The drawing under review shows one solid part. Ordinate dimensions are in mm from its lowest x, y, z. A direction names the side the tool comes from. Coordinates: 2 decimals unless noted, no trailing zeros. Write each loop counter-clockwise with the first axis right and the second up, starting at its lowest first coordinate (ties: lowest second). Pieces come first, ordered by that corner, then holes.
Q1. Insertion check: pin 1 (10 mm diameter, centred on x = 38.5, z = 21, fed in from -Y); pin 2 (6 mm diameter, centred on y = 11, z = 19.1, fed in from -X); pin 3 (4.5 mm diameter, centred on y = 79, z = 19.1, fed in from -X); pin 4 (4 mm diameter, centred on x = 94, z = 28.5, fed in from -Y). Each pin has a flat end and moves straight along its axis. Give the tip position at first contact, or say it passes through.
Q2. Take a section at D-D (y = 11). Give the boundary of the cut face in (x, z).
Q3. Take a section at A-A (y = 32). Give the boundary of the cut face in (x, z).
Q4. Mouldability with a two-part tool opening along X and no side actions: class the marked faces 3, 4 and 5 as pulls with the +X half, pulls with the -X half, needs draft (parallel to the pull), parting line crosses it, or undercut.
Q5. Take a section at C-C (z = 19.1). State how many separate pieces and enclosed holes the cut face has, and give its area (3 significant figures).
Q6. Take a section at B-B (x = 75). Give the boundary of the cut face in (y, z).
Q7. Machinability: for the marked faces 1 and 2, which of the approach directions +Z, -Z, +X, -X, +Y, -Y give a long, thin tool a straight path to every point of the face, cutting with its end or side? Answer none if there is none.
Q8. For probe 1 along X at (y, z) = (32, 17.5); probe 2 along Y at (x, z) = (2.3, 19.1); probe 3 along Y at (x, z) = (1, 19) (1 decimal), list the stretches that pass through material, from the lowest coordinate up.
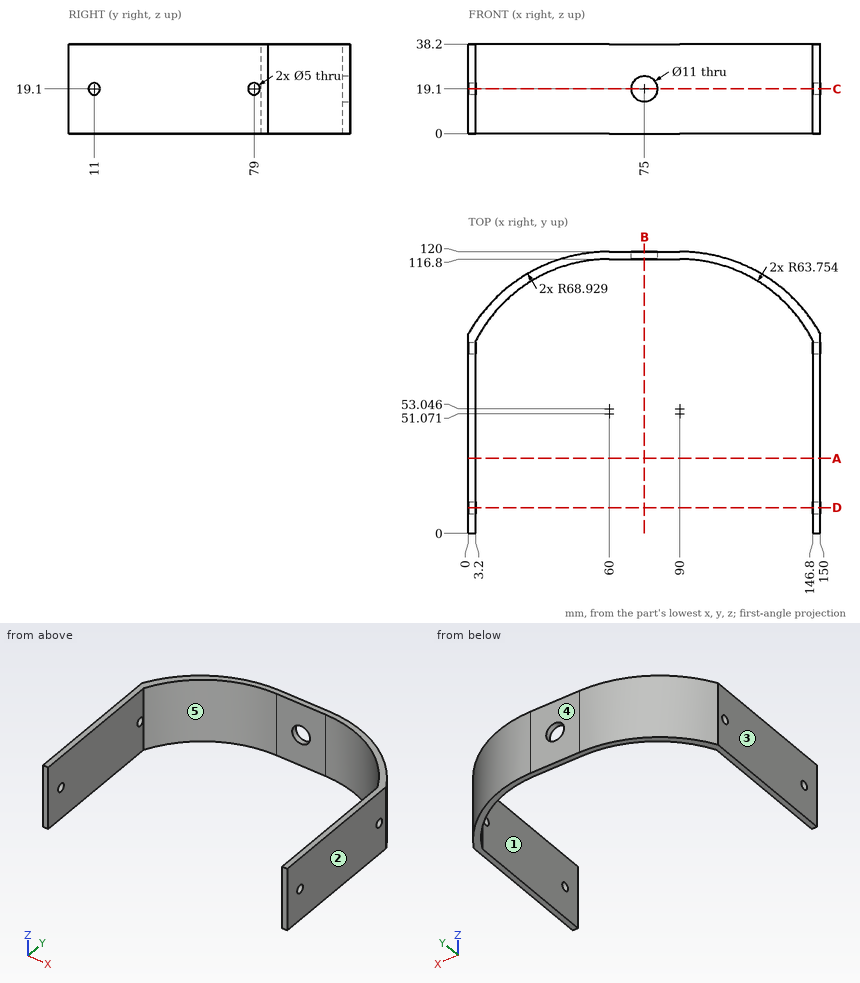
Response:
1. pin 1: stops at y = 111.03
1. pin 2: stops at x = 0
1. pin 3: passes through
1. pin 4: stops at y = 116.52
2. outline: (0, 0) - (3.2, 0) - (3.2, 16.6) - (0, 16.6) - close; (0, 21.6) - (3.2, 21.6) - (3.2, 38.2) - (0, 38.2) - close; (146.8, 0) - (150, 0) - (150, 16.6) - (146.8, 16.6) - close; (146.8, 21.6) - (150, 21.6) - (150, 38.2) - (146.8, 38.2) - close
3. outline: (0, 0) - (3.2, 0) - (3.2, 38.2) - (0, 38.2) - close; (146.8, 0) - (150, 0) - (150, 38.2) - (146.8, 38.2) - close
4. face 3: pulls with the -X half
4. face 4: needs draft
4. face 5: undercut
5. separate pieces: 6
5. enclosed holes: 0
5. area: 1,040 mm2
6. outline: (116.8, 0) - (120, 0) - (120, 13.6) - (116.8, 13.6) - close; (116.8, 24.6) - (120, 24.6) - (120, 38.2) - (116.8, 38.2) - close
7. face 1: +Z, -Z, -Y
7. face 2: +Z, -Z, +X, +Y, -Y
8. probe 1: x = 0 to 3.2, 146.8 to 150
8. probe 2: y = 0 to 8.5, 13.5 to 76.5, 81.5 to 88.78
8. probe 3: y = 0 to 8.5, 13.5 to 76.5, 81.5 to 86.7
